Source: CAD feature listing. Evaluate the final solid. Frame: model axes, mm. A direction names the side the tool comes from. Give positions to 0.01 mm unless a question says otherwise; leave off trailing zeros. Loops run counter-clockwise (first coordinate to the right, second up) from the corner with the lowest first, then second, coordinate; pieces in that order, holes last. Notation, with made-up numbers: (8.25, 52) -> (18.25, 52) arc R9 cw to (18.25, 67) -> close; hole circle Ø8 at (-16.75, 29.5). An arc over 180 degrees is marked (long way). Answer as a JSON object with one key per item and string values. Group by question number.
from build123d import *

# Parameters (mm, degrees)
F_3_8_0_375_DIAMETER_HOLE1_D           = 9.525
F_3_8_0_375_DIAMETER_HOLE1_DEPTH       = 13.335
F_3_8_0_375_DIAMETER_HOLE1_CSINK_D     = 10.16
F_3_8_0_375_DIAMETER_HOLE1_CSINK_ANGLE = 90
F_3_8_0_375_DIAMETER_HOLE1_TIP         = 2.861598698
SKETCH4_R                              = 1.27
CUT_EXTRUDE1_DEPTH                     = 29.323277935
CHAMFER1_SIZE                          = 1.524
CUT_EXTRUDE2_DEPTH                     = 42.076598545
CHAMFER2_SIZE                          = 1.27
SKETCH6_R                              = 6.604
SKETCH6_R_2                            = 6.35
CUT_EXTRUDE3_DEPTH                     = 0.254
CHAMFER3_SIZE                          = 0.762


with BuildPart() as part:
    # Sketch1 → Revolve1 (revolve)
    with BuildSketch(Plane.XY, mode=Mode.PRIVATE) as revolve1_sk:
        Polygon((9.525, 0), (14.224, 0), (14.224, 16.51), (8.89, 21.59), (8.89, 23.0378), (10.4394, 24.5872), (10.4394, 35.814), (0, 35.814), (0, 14.097), (1.27, 14.097), (1.27, 15.875), (9.525, 15.875), align=None)
    revolve(revolve1_sk.sketch.rotate(Axis((0, 1.826937735, 0), (0, 1, 0)), 90), axis=Axis((0, 1.826937735, 0), (0, 1, 0)))

    # 3/8 (0.375) Diameter Hole1
    with Locations(Plane(origin=(0, 35.814, 0), x_dir=(1, 0, 0), z_dir=(0, 1, 0))):
        with Locations((0, 0)):
            CounterSinkHole(F_3_8_0_375_DIAMETER_HOLE1_D / 2, F_3_8_0_375_DIAMETER_HOLE1_CSINK_D / 2, depth=F_3_8_0_375_DIAMETER_HOLE1_DEPTH, counter_sink_angle=F_3_8_0_375_DIAMETER_HOLE1_CSINK_ANGLE)
            with Locations((0, 0, -(F_3_8_0_375_DIAMETER_HOLE1_DEPTH + F_3_8_0_375_DIAMETER_HOLE1_TIP / 2))):  # 118° drill point
                Cone(0, F_3_8_0_375_DIAMETER_HOLE1_D / 2, F_3_8_0_375_DIAMETER_HOLE1_TIP, mode=Mode.SUBTRACT)

    # Sketch4 → Cut-Extrude1 (cut, through all)
    with BuildSketch(Plane.XZ.offset(-15.875)):
        with Locations(Location((2.54, 0, 0), (0, 0, 223.987874518))):
            Circle(SKETCH4_R)
    extrude(amount=-CUT_EXTRUDE1_DEPTH, mode=Mode.SUBTRACT)

    # Chamfer1
    chamfer1_edges = [part.edges().sort_by_distance(p)[0] for p in [
        (0, 0, 14.224),
    ]]
    chamfer(chamfer1_edges, length=CHAMFER1_SIZE)

    # Sketch5 → Cut-Extrude2 (cut, through all)
    with BuildSketch(Plane.XZ):
        with BuildLine():
            ThreePointArc((7.112, -12.318345343), (12.318345343, -7.112), (14.224, 0))
            Line((14.224, 0), (7.112, -12.318345343))
        make_face()
        with BuildLine():
            Line((7.112, 12.318345343), (14.224, 0))
            ThreePointArc((14.224, 0), (12.318345343, 7.112), (7.112, 12.318345343))
        make_face()
        with BuildLine():
            Line((-7.112, 12.318345343), (7.112, 12.318345343))
            ThreePointArc((7.112, 12.318345343), (0, 14.224), (-7.112, 12.318345343))
        make_face()
        with BuildLine():
            ThreePointArc((-7.112, -12.318345343), (0, -14.224), (7.112, -12.318345343))
            Line((7.112, -12.318345343), (-7.112, -12.318345343))
        make_face()
        with BuildLine():
            Line((-14.224, 0), (-7.112, 12.318345343))
            ThreePointArc((-7.112, 12.318345343), (-12.318345343, 7.112), (-14.224, 0))
        make_face()
        with BuildLine():
            ThreePointArc((-14.224, 0), (-12.318345343, -7.112), (-7.112, -12.318345343))
            Line((-7.112, -12.318345343), (-14.224, 0))
        make_face()
    extrude(amount=-CUT_EXTRUDE2_DEPTH, mode=Mode.SUBTRACT)

    # Chamfer2
    chamfer2_edges = [part.edges().sort_by_distance(p)[0] for p in [
        (0, 35.814, 10.4394),
    ]]
    chamfer(chamfer2_edges, length=CHAMFER2_SIZE)

    # Sketch6 → Cut-Extrude3 (cut)
    with BuildSketch(Plane(origin=(0, 35.814, 0), x_dir=(1, 0, 0), z_dir=(0, 1, 0))):
        with Locations(Location((0, 0, 0), (0, 0, 270))):
            Circle(SKETCH6_R)
        with Locations(Location((0, 0, 0), (0, 0, 270))):
            Circle(SKETCH6_R_2, mode=Mode.SUBTRACT)
    extrude(amount=-CUT_EXTRUDE3_DEPTH, mode=Mode.SUBTRACT)

    # Chamfer3
    chamfer3_edges = [part.edges().sort_by_distance(p)[0] for p in [
        (0, 0, 9.525),
    ]]
    chamfer(chamfer3_edges, length=CHAMFER3_SIZE)


solid = part.part
(1) Mould query, pull axis X, two halves, no side actions, for faces 1 (the face through (0, 15.875, 2)), 2 (the face through (6.611, 0.434, -11.349)), 3 (the face through (-10.7, 9, 6.1)). Classes: pulls with the +X half, pulls with the -X half, needs draft (parallel to the pull), parting line crosses it, or undercut.
(2) First-contact query: pin 1 (10.5 mm diameter, centred on x = 1, z = -1, fed in from +Y); pin 2 (4 mm diameter, centred on y = 23.5, z = 6, fed in from -X); pin 3 (1 mm diameter, centred on x = -9, z = -1.5, fed in from -Y); pin 4 (4 mm diameter, centred on x = 2.54, z = 0, fed in from +Y). Flat tips, straight axial feed; report the tip coordinate or a pass-through.
(3) Section query B-B on y = 27. Return the cut outline in (x, z) (1 decimal).
(4) Material intervals for line 1 (Z direction, x = 2.54, y = 17.75); line 2 (Z direction, x = -5.5, y = 7.5); line 3 (Y direction, x = 8, z = -3) (3 decimals), sorted ascending. Write a range as from..to.
(5) Access query for faces 4 (the face through (3.78, 28.9, 2.9)), 5 (the face through (0, 14.097, 0)), 6 (the face through (3.81, 18.85, 0.03)). Directions: +Z, -Z, +X, -X, +Y, -Y. A direction counts if a zero-diameter tool reaches every point of the face in a straight line with its end or side. Return the directions, or none.
(6) Section query A-A on y = 7. Return the cut outline in (x, z) (3 decimals).
Result:
{
 "1": {"face 1": "undercut", "face 2": "pulls with the +X half", "face 3": "pulls with the -X half"},
 "2": {"pin 1": "y = 35.81", "pin 2": "x = -9.5", "pin 3": "y = 0.66", "pin 4": "y = 22.35"},
 "3": {"outline": "circle Ø20.9 at (0, 0); hole circle Ø9.5 at (0, 0)"},
 "4": {"line 1": "-12.32..-1.27, 1.27..12.32", "line 2": "-12.32..-7.78, 7.78..12.32", "line 3": "15.875..35.814"},
 "5": {"face 4": "+Y", "face 5": "-Y", "face 6": "+Y, -Y"},
 "6": {"outline": "(-14.224, 0) -> (-7.112, -12.318) -> (7.112, -12.318) -> (14.224, 0) -> (7.112, 12.318) -> (-7.112, 12.318) -> close; hole circle Ø19.05 at (0, 0)"}
}
